The figure shows three views and two pictorial views of one solid part (mm, origin at its lowest corner). Answer the questions. A direction names the side the tool comes from. Give positions to 0.01 mm unless a question says otherwise; leave off trailing zeros. Order: outer loops, then holes, each group sorted by start corner. A loop starts at its lowest first (then second) coordinate and runs counter-clockwise, first axis right, second up. Notation, with made-up numbers: M 26.5,-22.75 L 31.5,-22.75 A30 cw 31.5,10.25 Z; hole C -4.5,40.25 d5. An arc over 180 degrees is marked long. One line per item, written item: value.
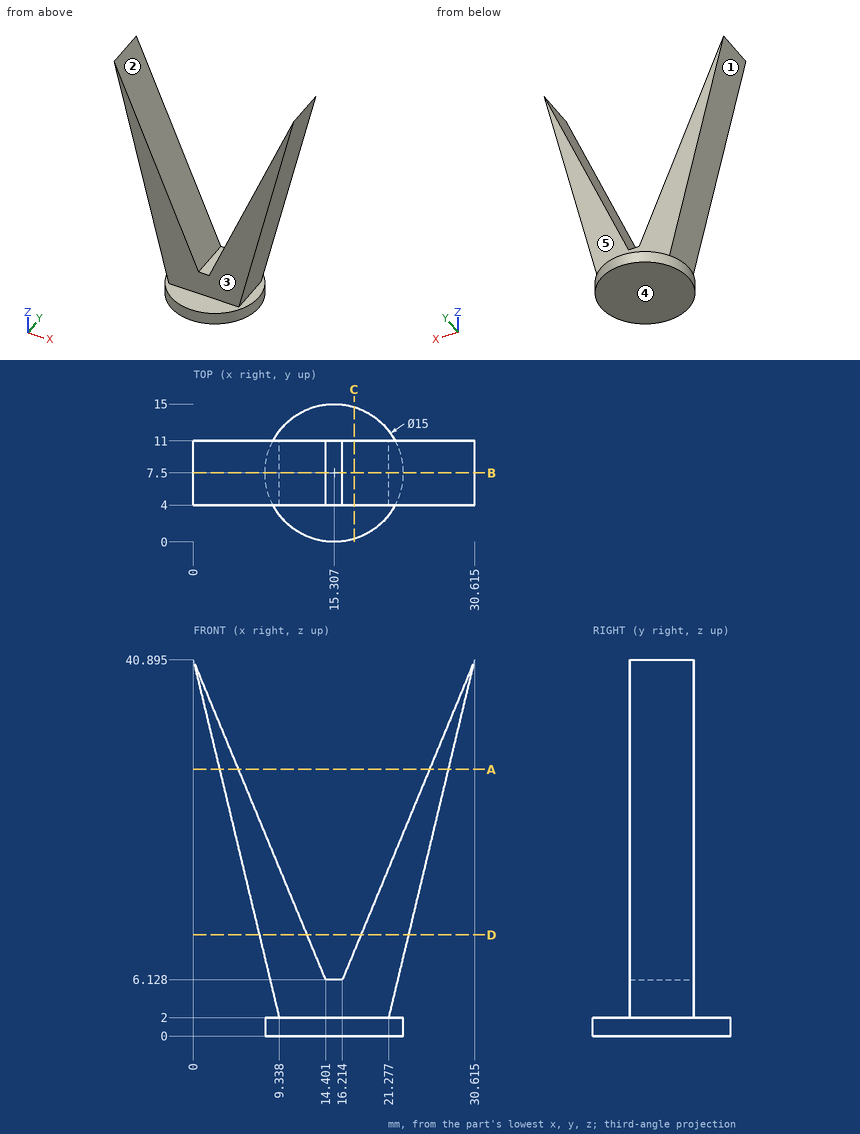
1) Determine the mould class of the marked faces 1, 2 and 3 for opening direction X: +X half, -X half, draft (parallel to the pull), parting line (faces both ways), or undercut.
Reported:
face 1: -X half
face 2: undercut
face 3: draft
2) Find section C-C, the plane x = 17.5. Write down the section's boundary in (y, z).
Reported:
outline: M 0.33,0 L 14.67,0 L 14.67,2 L 11,2 L 11,9.23 L 4,9.23 L 4,2 L 0.33,2 Z
3) Consider probe 1 along Y at (x, z) = (9, 4); probe 2 along Z at (x, y) = (14, 3.75); probe 3 along X at (y, z) = (9, 11.5) (1 decimal). Determine where each line is inside the solid, lowest interval first.
Reported:
probe 1: y = 4 to 11
probe 2: z = 0 to 2
probe 3: x = 7.1 to 12.2, 18.4 to 23.6
4) Which of the six approach directions +Z, -Z, +X, -X, +Y, -Y give full straight-line access (tool end or side, diameter ignored) to the marked faces 4 and 5?
Reported:
face 4: -Z, +X, -X, +Y, -Y
face 5: +Z, +X, -X, +Y
5) Find section B-B, the plane y = 7.5. Write down the section's boundary in (x, z) (1 decimal).
Reported:
outline: M 0,40.9 L 9.3,2 L 7.8,2 L 7.8,0 L 22.8,0 L 22.8,2 L 21.3,2 L 30.6,40.9 L 16.2,6.1 L 14.4,6.1 Z
6) Find section A-A, the plane z = 29. Write down the section's boundary in (x, y), plus the area to 3 significant figures.
Reported:
outline: M 2.86,4 L 4.93,4 L 4.93,11 L 2.86,11 Z; M 25.69,4 L 27.76,4 L 27.76,11 L 25.69,11 Z
area: 29.0 mm^2
7) Find section D-D, the plane z = 11. Write down the section's boundary in (x, y).
Reported:
outline: M 7.18,4 L 12.38,4 L 12.38,11 L 7.18,11 Z; M 18.23,4 L 23.44,4 L 23.44,11 L 18.23,11 Z
8) Each of these flat-tipped pins is pushed along its axis until it touches: pin 1 Ø4 at (y, z) = (12.5, 10.5) entering from -X; pin 2 Ø6 at (y, z) = (6, 16) entering from -X; pin 3 Ø6 at (x, z) = (9, 17.5) entering from -Y. Where does it stop, or does it pass through?
Reported:
pin 1: stops at x = 6.98
pin 2: stops at x = 5.26
pin 3: stops at y = 4
